Part print with two shaded views. Sizes in mm from the minimum x, y, z corner. A direction names the side the tool comes from. Round coordinates to 2 decimals unless told otherwise and drop trailing zeros. Write each loop counter-clockwise with the first axis right and the second up, starting at its lowest first coordinate (ties: lowest second). Pieces come first, ordered by that corner, then holes.
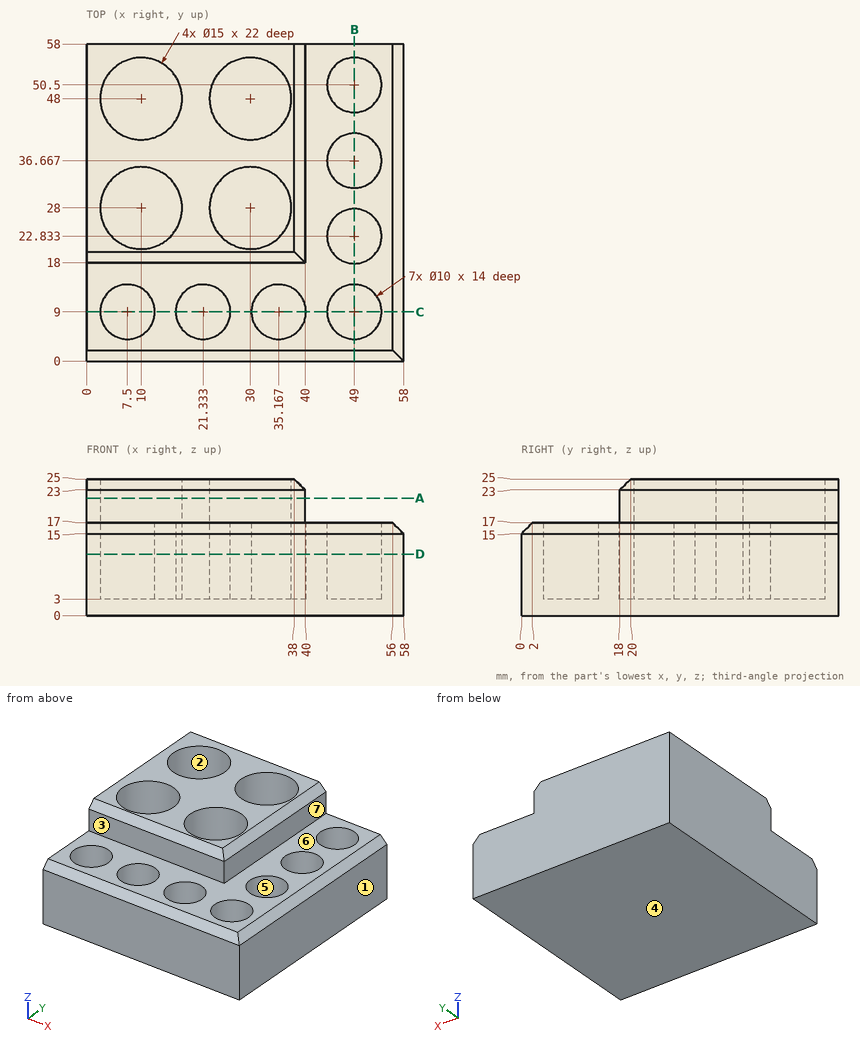
Q1. Cut at A-A on z = 21.5. Write the cut outline in (x, y), plus the area to 3 significant figures.
Values follow:
outline: (0, 18) - (40, 18) - (40, 58) - (0, 58) - close; hole circle Ø15 at (10, 28); hole circle Ø15 at (10, 48); hole circle Ø15 at (30, 28); hole circle Ø15 at (30, 48)
area: 893 mm2
Q2. Mould opens along Y. For the marked faces 1, 2 and 3 say: +Y half, -Y half, draft (parallel to the pull), parting line (faces both ways), or undercut.
Values follow:
face 1: draft
face 2: undercut
face 3: -Y half
Q3. Wall check: L1, parallel to Y at x = 49, z = 13.5; L2, parallel to X at y = 10, z = 7 (1 decimal); L3, parallel to Y at x = 24.5, z = 24. Give the ranges that are in metal, low to high.
Values follow:
L1: y = 0 to 4, 14 to 17.83, 27.83 to 31.67, 41.67 to 45.5, 55.5 to 58
L2: x = 0 to 2.6, 12.4 to 16.4, 26.2 to 30.3, 40.1 to 44.1, 53.9 to 58
L3: y = 19 to 22.9, 33.1 to 42.9, 53.1 to 58
Q4. Drop flat-ended pins along their axis: pin 1 (4.5 mm diameter, centred on x = 13.5, y = 27.5, fed in from +Z); pin 2 (5 mm diameter, centred on x = 50.5, z = 19, fed in from -Y); pin 3 (1.8 mm diameter, centred on x = 21.5, z = 21, fed in from -Y). Give the stop position or say it passes through.
Values follow:
pin 1: stops at z = 3
pin 2: stops at y = 1.5
pin 3: stops at y = 18
Q5. Cut at D-D on z = 11.25. State how many separate pieces and enclosed holes the cut face has, plus the area to 3 significant figures.
Values follow:
separate pieces: 1
enclosed holes: 11
area: 2,110 mm2
Q6. Cut at C-C on y = 9. Write the cut outline in (x, z), plus the area to 3 significant figures.
Values follow:
outline: (0, 0) - (58, 0) - (58, 15) - (56, 17) - (54, 17) - (54, 3) - (44, 3) - (44, 17) - (40.17, 17) - (40.17, 3) - (30.17, 3) - (30.17, 17) - (26.33, 17) - (26.33, 3) - (16.33, 3) - (16.33, 17) - (12.5, 17) - (12.5, 3) - (2.5, 3) - (2.5, 17) - (0, 17) - close
area: 424 mm2
Q7. Which spindle directions (+Z, -Z, +X, -X, +Y, -Y) get a long thin tool onto all of the face, cutting with end or side? Do the marked faces 4, 5, 6 and 7. Say none if no direction does.
Values follow:
face 4: -Z, +X, -X, +Y, -Y
face 5: +Z
face 6: +Z, +X, -Y
face 7: +Z, +X, +Y, -Y
Q8. Cut at B-B on x = 49. Write the cut outline in (y, z), plus the area to 3 significant figures.
Values follow:
outline: (0, 0) - (58, 0) - (58, 17) - (55.5, 17) - (55.5, 3) - (45.5, 3) - (45.5, 17) - (41.67, 17) - (41.67, 3) - (31.67, 3) - (31.67, 17) - (27.83, 17) - (27.83, 3) - (17.83, 3) - (17.83, 17) - (14, 17) - (14, 3) - (4, 3) - (4, 17) - (2, 17) - (0, 15) - close
area: 424 mm2
